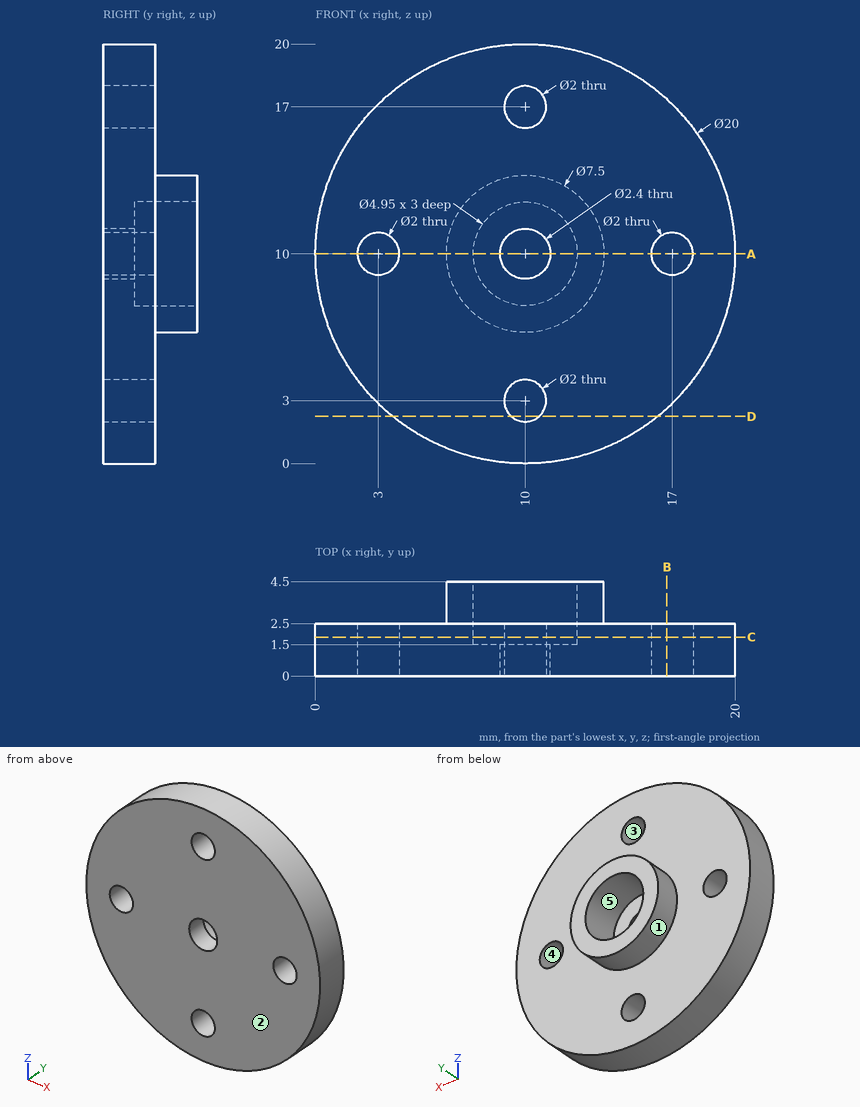
Study the drawing (mm; zero at the part's minimum x, y, z) and answer. A direction names the side the tool comes from. Give positions to 0.01 mm unless a question says otherwise; leave off trailing zeros. Order: outer loops, then holes, each group sorted by start corner. A loop starts at its lowest first (then second) coordinate and runs counter-clockwise, first axis right, second up. Notation, with made-up numbers: M 37.25,85 L 43.25,85 A20 cw 43.25,118 Z; hole C -36.5,-36.75 d5. An arc over 180 degrees is marked long. Put each result on its own line as item: value. Start each with the question number.
Item 1: For a pull along Z with two mould halves and no side action, classify the marked faces 1, 2 and 3 as +Z half, -Z half, draft (parallel to the pull), parting line (faces both ways), or undercut.
Item 2: The part is cut by section D-D, the plane z = 2.25. Determine the outline of the cut face in (x, y), and give its area (3 significant figures).
Item 3: Find the intervals of material crossed by line 1 along X through (y, z) = (0.8, 10); line 2 along X through (y, z) = (1.75, 10) (3 decimals); line 3 along X through (y, z) = (3.55, 10) (3 decimals), in increasing order.
Item 4: The part is cut by section B-B, the plane x = 16.75. Determine the outline of the cut face in (y, z), and give its area (3 significant figures).
Item 5: A flat-ended cylindrical pin translates along its axis: P1, Ø1.2, axis at x = 17, z = 10, coming from the -Y side. Find the tip coordinate at first contact, or state that the pin passes through.
Item 6: Which of the six approach directions +Z, -Z, +X, -X, +Y, -Y give full straight-line access (tool end or side, diameter ignored) to the marked faces 4 and 5?
Item 7: The part is cut by section A-A, the plane z = 10. Determine the outline of the cut face in (x, y) (3 decimals), and give its area (4 significant figures).
Item 8: The part is cut by section C-C, the plane y = 1.85. Determine the outline of the cut face in (x, z) (3 decimals), and give its area (3 significant figures).
Answer key:
1. face 1: parting line
1. face 2: draft
1. face 3: undercut
2. outline: M 3.68,0 L 9.34,0 L 9.34,2.5 L 3.68,2.5 Z; M 10.66,0 L 16.32,0 L 16.32,2.5 L 10.66,2.5 Z
2. area: 28.3 mm²
3. line 1: x = 0 to 2, 4 to 8.8, 11.2 to 16, 18 to 20
3. line 2: x = 0 to 2, 4 to 7.525, 12.475 to 16, 18 to 20
3. line 3: x = 6.25 to 7.525, 12.475 to 13.75
4. outline: M 0,2.62 L 2.5,2.62 L 2.5,9.03 L 0,9.03 Z; M 0,10.97 L 2.5,10.97 L 2.5,17.38 L 0,17.38 Z
4. area: 32.0 mm²
5. P1: passes through
6. face 4: +Y, -Y
6. face 5: +Y
7. outline: M 0,0 L 2,0 L 2,2.5 L 0,2.5 Z; M 4,0 L 8.8,0 L 8.8,1.5 L 7.525,1.5 L 7.525,4.5 L 6.25,4.5 L 6.25,2.5 L 4,2.5 Z; M 11.2,0 L 16,0 L 16,2.5 L 13.75,2.5 L 13.75,4.5 L 12.475,4.5 L 12.475,1.5 L 11.2,1.5 Z; M 18,0 L 20,0 L 20,2.5 L 18,2.5 Z
7. area: 36.55 mm²
8. outline: C 10,10 d20; hole C 3,10 d2; hole C 10,10 d4.95; hole C 10,3 d2; hole C 10,17 d2; hole C 17,10 d2
8. area: 282 mm²
